Can you work these out from the model? Positions are in its coordinate system, mm. A direction names the side the tool comes from. Coordinates: 2 decimals unless noted, no trailing zeros. Loops run counter-clockwise (first coordinate to the right, second up) from the corner with the lowest first, then second, coordinate; pieces in that order, holes last.
```python
from build123d import *

# Parameters (mm, degrees)
SKETCH1_R                      = 5.1
BASE_FLANGE1_DEPTH             = 2.8
EDGE_FLANGE1_STRIP_W           = 13.2
EDGE_FLANGE1_STRIP_H           = 2.8
EDGE_FLANGE1_STRIP_CUT_DEPTH   = 50
EDGE_FLANGE1_STRIP_2_W         = 13.2
EDGE_FLANGE1_STRIP_2_H         = 2.8
EDGE_FLANGE1_STRIP_CUT_2_DEPTH = 50
EDGE_FLANGE1_DEPTH             = 50
EDGE_FLANGE1_BEND_DEPTH        = 50
EDGE_FLANGE2_START             = -25
EDGE_FLANGE2_DEPTH             = 50
EDGE_FLANGE2_2_DEPTH           = 50
SKETCH20_R                     = 3.15
CUT_EXTRUDE1_DEPTH             = 72.206525832
FILLET1_R                      = 10
FILLET2_R                      = 2


# Read off the part's stored shape, not the designer's step: Edge-Flange2
# Sheet-metal steps are written as plain solids
with BuildPart() as part:
    # Sketch1 → Base-Flange1 (new body)
    with BuildSketch(Plane(origin=(0, 0, 0), x_dir=(1, 0, 0), z_dir=(0, 1, 0))):
        Polygon((-25, 29), (25, 29), (25, 10), (45, 10), (45, -10), (25, -10), (25, -29), (-25, -29), (-25, -10), (-45, -10), (-45, 10), (-25, 10), align=None)
        with Locations(Location((-35, 0, 0), (0, 0, 270))):
            Circle(SKETCH1_R, mode=Mode.SUBTRACT)
        with BuildLine():
            Line((32.5, 5.15), (37.5, 5.15))
            ThreePointArc((37.5, 5.15), (42.65, 0), (37.5, -5.15))
            Line((37.5, -5.15), (32.5, -5.15))
            ThreePointArc((32.5, -5.15), (27.35, 0), (32.5, 5.15))
        make_face(mode=Mode.SUBTRACT)
    extrude(amount=-BASE_FLANGE1_DEPTH)

    # Edge-Flange1 strip (across the edge) → Edge-Flange1 strip cut (cut)
    with BuildSketch(Plane(origin=(25, 0, -29), x_dir=(0, 0, 1), z_dir=(-1, 0, 0))):
        with Locations((-2.8, -1.4)):
            Rectangle(EDGE_FLANGE1_STRIP_W, EDGE_FLANGE1_STRIP_H)
    extrude(amount=EDGE_FLANGE1_STRIP_CUT_DEPTH, mode=Mode.SUBTRACT)

    # Edge-Flange1 strip 2 (across the edge) → Edge-Flange1 strip cut 2 (cut)
    with BuildSketch(Plane(origin=(-25, 0, 29), x_dir=(0, 0, -1), z_dir=(1, 0, 0))):
        with Locations((-2.8, -1.4)):
            Rectangle(EDGE_FLANGE1_STRIP_2_W, EDGE_FLANGE1_STRIP_2_H)
    extrude(amount=EDGE_FLANGE1_STRIP_CUT_2_DEPTH, mode=Mode.SUBTRACT)

    # Edge-Flange1 section (across the edge) → Edge-Flange1 (add)
    with BuildSketch(Plane(origin=(25, 0, -29), x_dir=(0, 0, 1), z_dir=(-1, 0, 0))):
        with BuildLine():
            Line((0, 1), (0, 37.2))
            Line((0, 37.2), (2.8, 37.2))
            Line((2.8, 37.2), (2.8, 1))
            ThreePointArc((2.8, 1), (3.092893219, 0.292893219), (3.8, 0))
            Line((3.8, 0), (3.8, -2.8))
            ThreePointArc((3.8, -2.8), (1.112994231, -1.687005769), (0, 1))
        make_face()
    extrude(amount=EDGE_FLANGE1_DEPTH)

    # Edge-Flange1 section 2 (across the edge) → Edge-Flange1 bend (add)
    with BuildSketch(Plane(origin=(-25, 0, 29), x_dir=(0, 0, -1), z_dir=(1, 0, 0))):
        with BuildLine():
            Line((0, 1), (0, 37.2))
            Line((0, 37.2), (2.8, 37.2))
            Line((2.8, 37.2), (2.8, 1))
            ThreePointArc((2.8, 1), (3.092893219, 0.292893219), (3.8, 0))
            Line((3.8, 0), (3.8, -2.8))
            ThreePointArc((3.8, -2.8), (1.112994231, -1.687005769), (0, 1))
        make_face()
    extrude(amount=EDGE_FLANGE1_BEND_DEPTH)

    # Edge-Flange2 outline → Edge-Flange2 (cut)
    with BuildSketch(Plane.YZ.offset(EDGE_FLANGE2_START)):
        with BuildLine():
            ThreePointArc((32.661988168, -26.2), (33.790654641, -26.399014351), (34.78318728, -26.972053338))
            Line((34.78318728, -26.972053338), (37.2, -29))
            Line((37.2, -29), (37.2, -26.2))
            Line((37.2, -26.2), (32.661988168, -26.2))
        make_face()
        with BuildLine():
            Line((37.2, 29), (34.78318728, 26.972053338))
            ThreePointArc((34.78318728, 26.972053338), (33.790654641, 26.399014351), (32.661988168, 26.2))
            Line((32.661988168, 26.2), (37.2, 26.2))
            Line((37.2, 26.2), (37.2, 29))
        make_face()
    extrude(amount=EDGE_FLANGE2_DEPTH, mode=Mode.SUBTRACT)

    # Edge-Flange2 2 outline → Edge-Flange2 2 (add)
    with BuildSketch(Plane.YZ.offset(EDGE_FLANGE2_START)):
        with BuildLine():
            Line((42.289578815, -33.270663707), (37.2, -29))
            Line((37.2, -29), (32.661988168, -29))
            ThreePointArc((32.661988168, -29), (32.832998239, -29.03015369), (32.983381973, -29.116977778))
            Line((32.983381973, -29.116977778), (40.489773508, -35.415588147))
            Line((40.489773508, -35.415588147), (42.289578815, -33.270663707))
        make_face()
        with BuildLine():
            Line((32.661988168, 29), (37.2, 29))
            Line((37.2, 29), (42.289578815, 33.270663707))
            Line((42.289578815, 33.270663707), (40.489773508, 35.415588147))
            Line((40.489773508, 35.415588147), (32.983381973, 29.116977778))
            ThreePointArc((32.983381973, 29.116977778), (32.832998239, 29.03015369), (32.661988168, 29))
        make_face()
    extrude(amount=EDGE_FLANGE2_2_DEPTH)

    # Sketch20 → Cut-Extrude1 (cut, through all)
    with BuildSketch(Plane(origin=(0, 1.090431477, 1.29952563), x_dir=(1, 0, 0), z_dir=(0, 0.642787609686538, 0.7660444431189792))):
        with Locations(Location((-10, 49.78166725, 0), (0, 0, 270))):
            Circle(SKETCH20_R)
        with Locations(Location((10, 49.78166725, 0), (0, 0, 270))):
            Circle(SKETCH20_R)
    cut_extrude1 = extrude(amount=-CUT_EXTRUDE1_DEPTH, mode=Mode.SUBTRACT)

    # Mirror2: Cut-Extrude1 across plane
    add(cut_extrude1.mirror(Plane.XY), mode=Mode.SUBTRACT)

    # Fillet1
    # the kernel refuses this fillet: 10 mm, written as the material it takes off along each edge
    with BuildSketch(Plane(origin=(45, 25, -10), x_dir=(0, 0, 1), z_dir=(0, -1, 0)), Plane(origin=(45, 25, 10), x_dir=(-1, 0, 0), z_dir=(0, -1, 0)), Plane(origin=(-45, 25, -10), x_dir=(1, 0, 0), z_dir=(0, -1, 0)), Plane(origin=(-45, 25, 10), x_dir=(0, 0, -1), z_dir=(0, -1, 0))) as fillet1_piece_1:
        with BuildLine():
            CenterArc((FILLET1_R, FILLET1_R), FILLET1_R, 180, 90)
            Line((0, FILLET1_R), (0, 0))
            Line((0, 0), (FILLET1_R, 0))
        make_face()
    extrude(amount=52.8, mode=Mode.SUBTRACT)
    with BuildSketch(Plane(origin=(-25, 58.35926906, 14.119552631), x_dir=(0, -0.7660444430323039, -0.6427876097898334), z_dir=(0, -0.6427876097898335, 0.766044443032304)), Plane(origin=(25, 24.420083263, -54.566699223), x_dir=(-1, 0, 0), z_dir=(0, 0.6427876097898335, 0.766044443032304)), Plane(origin=(-25, 24.420083263, -54.566699223), x_dir=(0, -0.7660444430323039, 0.6427876097898334), z_dir=(0, 0.6427876097898335, 0.766044443032304))) as fillet1_piece_2:
        with BuildLine():
            CenterArc((FILLET1_R, FILLET1_R), FILLET1_R, 180, 90)
            Line((0, FILLET1_R), (0, 0))
            Line((0, 0), (FILLET1_R, 0))
        make_face()
    extrude(amount=52.799999999, mode=Mode.SUBTRACT)
    with BuildSketch(Plane(origin=(25, 58.35926906, 14.119552631), x_dir=(0, -0.766044443032304, -0.6427876097898335), z_dir=(0, -0.6427876097898335, 0.766044443032304))) as fillet1_piece_3:
        with BuildLine():
            CenterArc((FILLET1_R, -FILLET1_R), FILLET1_R, 90, 90)
            Line((0, -FILLET1_R), (0, 0))
            Line((0, 0), (FILLET1_R, 0))
        make_face()
    extrude(amount=52.799999999, mode=Mode.SUBTRACT)

    # Fillet2
    fillet2_edges = [part.edges().sort_by_distance(p)[0] for p in [
        (-25, -1.4, 10),
        (-25, -1.4, -10),
        (25, -1.4, -10),
        (25, -1.4, 10),
    ]]
    fillet(fillet2_edges, radius=FILLET2_R)


solid = part.part
```
(1) If we mould it in two halves opening along X, with no side actions, what happens to faces 1 (the cylindrical face through (-21.993, 39.204, 32.511)), 2 (the flat face through (-31, -1, 10)), 3 (the cylindrical face through (10.946, 36.036, 29.826)), 4 (the cylindrical face through (25.57, -1.42, -10.6))? For each: released by +X, released by -X, zero draft, split by the parting line, or undercut.
Check values:
face 1: released by -X
face 2: zero draft
face 3: undercut
face 4: released by +X
(2) Which directions (+Z, -Z, +X, -X, +Y, -Y) give clear straight access to the entire face, cutting with the end or side of a thin tool? Please do faces 5 (the flat face through (0, 17, -26.2)), 6 (the cylindrical face through (27.35, -1.38, 0.11)), 7 (the flat face through (0, 17, -29)), 8 (the flat face through (31, -1, 10)).
Check values:
face 5: +X, -X, +Y
face 6: +Y, -Y
face 7: -Z, +X, -X, -Y
face 8: +Z, +X, +Y, -Y
(3) I'm going to push flat-ended pins straight in: pin 1 (2 mm diameter, centred on x = 35.5, y = -1, fed in from +Z); pin 2 (6 mm diameter, centred on y = 2, z = -18.5, fed in from +X); pin 3 (1.4 mm diameter, centred on x = -30, y = -2, fed in from -Z); pin 4 (11.5 mm diameter, centred on x = -35, z = 0, fed in from -Y). Where does each tip first touch, or does it pass through?
Check values:
pin 1: stops at z = 10
pin 2: stops at x = 25
pin 3: stops at z = -10
pin 4: stops at y = -2.8
(4) I want a section at D-D on x = 31.5. Write out the boundary of the cut face in (y, z).
Check values:
outline: (-2.8, -10) - (0, -10) - (0, -5.05) - (-2.8, -5.05) - close; (-2.8, 5.05) - (0, 5.05) - (0, 10) - (-2.8, 10) - close
(5) I want a section at C-C on y = 16.5. Write out the boundary of the cut face in (x, z).
Check values:
outline: (-25, -29) - (25, -29) - (25, -26.2) - (-25, -26.2) - close; (-25, 26.2) - (25, 26.2) - (25, 29) - (-25, 29) - close
(6) I want a section at A-A on z = 0. Write out the boundary of the cut face in (x, y), then the cut area to 3 significant figures.
Check values:
outline: (-45, -2.8) - (-40.1, -2.8) - (-40.1, 0) - (-45, 0) - close; (-29.9, -2.8) - (27.35, -2.8) - (27.35, 0) - (-29.9, 0) - close; (42.65, -2.8) - (45, -2.8) - (45, 0) - (42.65, 0) - close
area: 181 mm2
(7) I want a section at B-B on x = -2. Write out the boundary of the cut face in (y, z).
Check values:
outline: (-2.8, -25.2) arc R3.8 ccw to (1, -29) - (32.66, -29) arc R0.5 cw to (32.98, -29.12) - (40.49, -35.42) - (42.29, -33.27) - (34.78, -26.97) arc R3.3 ccw to (32.66, -26.2) - (1, -26.2) arc R1 cw to (0, -25.2) - (0, 25.2) arc R1 cw to (1, 26.2) - (32.66, 26.2) arc R3.3 ccw to (34.78, 26.97) - (42.29, 33.27) - (40.49, 35.42) - (32.98, 29.12) arc R0.5 cw to (32.66, 29) - (1, 29) arc R3.8 ccw to (-2.8, 25.2) - close
(8) If I drill on probe 1 along X at (y, z) = (-1, 0); probe 2 along Z at (x, y) = (-11, 30); probe 3 along Z at (x, y) = (-14, 33), over which ranges is the centre line in solid material (lowest first)?
Check values:
probe 1: x = -45 to -40.1, -29.9 to 27.35, 42.65 to 45
probe 2: z = -29 to -26.2, 26.2 to 29
probe 3: z = -29.13 to -26.22, 26.22 to 29.13
